Input: part model. Units: mm. Frame: model coordinates. A direction names the side the tool comes from. Give positions to 0.01 mm unless a question says otherwise; leave off trailing zeros. Order: outer loops, then holes, each group sorted by start corner. A loop starts at its lowest first (then second) coordinate and runs counter-clockwise, first axis right, second up. Notation, with made-up numbers: (44.5, 64.5) - (103.5, 64.5) arc R20 ccw to (103.5, 82.5) - close; hole circle Ø9 at (-19, -28.5). An arc over 180 degrees is marked (long way). Answer in a Markdown table with one row per item. Add a question column.
1. Section query B-B on x = 7.5. Return loops of the section in (y, z), and give its area (3 significant figures).
2. Contact query for flat-ended pins moving along their axis: pin 1 (4 mm diameter, centred on x = -0.5, z = 2.5, fed in from -Y); pin 2 (5 mm diameter, centred on x = 30, y = 8, fed in from +Z); pin 3 (3 mm diameter, centred on x = 0.5, z = -5, fed in from -Y). Output: stop coordinate, or through.
3. Access query for faces 1 (the face through (0, -7, 0)), 2 (the face through (-4, 0, 9)). Directions: +Z, -Z, +X, -X, +Y, -Y. A direction counts if a zero-diameter tool reaches every point of the face in a straight line with its end or side. Return the directions, or none.
4. Ray query, line 1 (X direction, y = 3.25, z = -8); line 2 (Y direction, x = 19, z = 1.25); line 3 (Z direction, x = 11.5, y = -0.75). Return the intervals inside material, ascending. Write a range as [from, to].
5. Section query A-A on x = -2.5. Return loops of the section in (y, z), and give its area (3 significant figures).
Autodesk Inventor part; units mm, degrees
ref_plane "Work Plane1" through (1.525, 0, 0) normal (0, 0, 1) x (1, 0, 0)
ref_plane "YZ Plane" through (0, 0, 0) normal (1, 0, 0) x (0, 1, 0)
ref_plane "XZ Plane" through (0, 0, 0) normal (0, 1, 0) x (-1, 0, 0)
sketch "Skizze1" plane through (0, 0, 0) normal (0, 0, 1) x (1, 0, 0)
  line L0 (0, 6) -> (35, 6)
  line L1 (35, 6) -> (35, 0)
  line L2 (35, 0) -> (0, 0)
  line L3 (-7, 0) -> (42, 0)
  line L4 (0, -1.2) -> (0, 7.2)
  line L5 (0, 6) -> (0, 0)
  dimension "d2" = 12
  dimension "d59" = 35
revolve "Körper" add sketch "Skizze1" angle 360 about axis through (35, 0, 0) along (-1, 0, 0)
sketch "Skizze2" plane through (0, 0, 0) normal (-1, 0, 0) x (0, 0, 1)
  line L0 (0, 10.3923) -> (9, 5.1962)
  line L1 (9, 5.1962) -> (9, -5.1962)
  line L2 (9, -5.1962) -> (0, -10.3923)
  line L3 (0, -10.3923) -> (-9, -5.1962)
  line L4 (-9, -5.1962) -> (-9, 5.1962)
  line L5 (-9, 5.1962) -> (0, 10.3923)
  line L6 (-12.6, 0) -> (12.6, 0)
  line L7 (0, 14.5492) -> (0, -14.5492)
  point P0 (0, 0)
  point P1 (0, 0)
  dimension "d11" = 18
extrude "Kopf" add sketch "Skizze2" along normal blind 8
sketch "Skizze4" plane through (0, 0, 0) normal (0, 0, 1) x (1, 0, 0)
  line L0 (-6.9608, 10.8) -> (-8, 9)
  line L1 (-1.1, 0) -> (-0.234, 0)
  line L2 (-9.5532, 0) -> (1.3192, 0)
  line L3 (-8, 10.8) -> (-6.9608, 10.8)
  line L4 (-8, 9) -> (-8, 10.8)
  line L5 (0, 12.96) -> (0, -2.16)
  dimension "d65" = 18
  dimension "d67" = 30
  dimension "d68" = 21.6
  dimension "d69" = 8
revolve "Fase1" cut sketch "Skizze4" angle 360 about axis through (-1.1, 0, 0) along (1, 0, 0)
thread "Gewinde"
chamfer "Fase2" distance 1.0735 distance2 1.0736 1 edges at (35, -6, 0) measured on face at (35, -1.5551, -0.8476)
fillet "Fillet2" radius 0.6 1 edges at (0, -6, 0)
ref_plane "Work Plane1" through (1.525, 0, 0) normal (0, 0, 1) x (1, 0, 0)
equation "\"d71\" = RR"
equation "\"d11\" = SW"
equation "\"d3\" = KOH"
equation "\"d6\" = -0.5 * SPD + 0.5 * GD"
equation "\"d15\" = GEL"
equation "\"d2\" = GD"
equation "\"d59\" = NLG"
equation "\"d65\" = SW"
equation "\"d67\" = ANG1"
equation "\"d68\" = 1.2 * SW"
equation "\"d69\" = KOH"
equation "\"NLG\" = 35"
equation "\"GD\" = NND"
equation "\"BDM\" = NND"
equation "\"KOH\" = 8"
equation "\"GEL\" = 20.5"
equation "\"SW\" = 18"
equation "\"SW0\" = SW"
equation "\"SPD\" = NND - 1.2269 * PTC"
equation "\"SD2\" = NND"
equation "\"SD\" = 0"
equation "\"ANG1\" = 30deg"
equation "\"GAL\" = 0.61345 * PTC"
equation "\"GUL\" = 0.61345 * PTC"
equation "\"RR\" = 0.6"
equation "\"RR1\" = 0.1"
equation "\"GD1\" = THREADDIA - 1.2269 * PTC"
equation "\"THREADDIA\" = 12"
equation "\"SDH\" = NND"
equation "\"TOA\" = 30deg"
equation "\"PTC\" = 1.75"
equation "\"NND\" = 12"
equation "\"E0\" = 1.155 * SW"
equation "\"K1\" = 5.28"
properties part number "DIN 7990 - M12 x 35" material "Stahl, weich"
Answer:
| question | item | result |
|---|---|---|
| 1 | outline | circle Ø12 at (0, 0) |
| 1 | area | 113 mm² |
| 2 | pin 1 | stops at y = -10.1 |
| 2 | pin 2 | stops at z = 2.4 |
| 2 | pin 3 | stops at y = -8.32 |
| 3 | face 1 | +X |
| 3 | face 2 | +Z, +X, -X, +Y, -Y |
| 4 | line 1 | x = [-8, 0] |
| 4 | line 2 | y = [-5.87, 5.87] |
| 4 | line 3 | z = [-5.95, 5.95] |
| 5 | outline | (-10.39, 0) - (-5.2, -9) - (5.2, -9) - (10.39, 0) - (5.2, 9) - (-5.2, 9) - close |
| 5 | area | 281 mm² |
